```python
from build123d import *

# Parameters (mm, degrees)
F0_W     = 82.55
F0_H     = 355.6
F1_DEPTH = 4.7625
F3_D     = 9.525
F4_D     = 3
F5_D     = 6
F7_DEPTH = 4.7625


with BuildPart() as f1:
    # F0 (on Top) → F1 (new body)
    with BuildSketch(Plane.XY):
        with Locations((41.275, 0)):
            Rectangle(F0_W, F0_H)
        Polygon((82.55, 177.8), (82.55, -177.8), (139.7, -177.8), align=None)
        with Locations((-41.275, 0)):
            Rectangle(F0_W, F0_H)
        Polygon((-139.7, -177.8), (-82.55, -177.8), (-82.55, 177.8), align=None)
    extrude(amount=F1_DEPTH)

    # F3 (through all)
    with Locations(Plane.XY.offset(4.7625)):
        with Locations((-53.975, 67.945), (0, 121.92), (53.975, 67.945), (0, 13.97)):
            Hole(F3_D / 2)

    # F4 (through all)
    with Locations(Plane.XY.offset(4.7625)):
        with Locations((15.5, 83.445), (-15.5, 83.445), (-15.5, 52.445), (15.5, 52.445)):
            Hole(F4_D / 2)

    # F5 (through all)
    with Locations(Plane.XY.offset(4.7625)):
        with Locations((0, 67.945)):
            Hole(F5_D / 2)

    # F6 (on face) → F7 (join)
    with BuildSketch(Plane.XY.offset(4.7625)):
        with BuildLine():
            Line((-82.55, 177.8), (82.55, 177.8))
            ThreePointArc((82.55, 177.8), (0, 205.359059), (-82.55, 177.8))
        make_face()
    extrude(amount=-F7_DEPTH)


solid = f1.part
```
The model under review builds one solid part; all positions refer to its coordinate system, in mm. Give positions to 0.01 mm unless a question says otherwise; leave off trailing zeros. Write each loop counter-clockwise with the first axis right and the second up, starting at its lowest first coordinate (ties: lowest second). Pieces come first, ordered by that corner, then holes. Notation, with made-up numbers: M -30.75,-24 L -11.75,-24 A27 cw -11.75,-3 Z; hole C 45.5,66 d8. An arc over 180 degrees is marked long. Write item = value, one per line. Start each with the question number.
Q1. For line 1 (Y direction, x = 0, z = 1.25) (1 decimal); line 2 (Y direction, x = 15.5, z = 1.05) (3 decimals); line 3 (X direction, y = 16, z = 4.6), list the stretches that pass through material, from the lowest coordinate up.
Q2. We need section A-A (y = 13.97). State the section outline as (x, z) points.
Q3. We need section D-D (y = 121.92). State the section outline as (x, z) points.
Q4. Clearance check with a flat-ended pin moving along its axis: pin 1 (2 mm diameter, centred on y = -79.5, z = 2.5, fed in from +X). State where the tip first meets the part, or that it passes through.
Q5. We need section C-C (x = 94). State the section outline as (y, z) points, plus the area to 3 significant figures.
Q6. We need section B-B (z = 2.2). Give the number of separate pieces and of enclosed holes in the cut face, plus the area to 3 significant figures.
Q7. Mouldability with a two-part tool opening along Y and no side actions: class faces 1 (the face through (-2, -26, 0)), 2 (the face through (3.5, 17.2, 2.3)), 3 (the face through (1.24, 205.353, 2.415)) as released by +Y, released by -Y, zero draft, split by the parting line, or undercut.
Result set:
q1.line_1 = -177.8 to 9.2, 18.7 to 64.9, 70.9 to 117.2, 126.7 to 205.4
q1.line_2 = -177.8 to 50.945, 53.945 to 81.945, 84.945 to 204.482
q1.line_3 = -108.55 to -4.31, 4.31 to 108.55
q2.outline = M -108.88,0 L -4.76,0 L -4.76,4.76 L -108.88,4.76 Z; M 4.76,0 L 108.88,0 L 108.88,4.76 L 4.76,4.76 Z
q3.outline = M -91.53,0 L -4.76,0 L -4.76,4.76 L -91.53,4.76 Z; M 4.76,0 L 91.53,0 L 91.53,4.76 L 4.76,4.76 Z
q4.pin_1 = 124.06
q5.outline = M -177.8,0 L 106.56,0 L 106.56,4.76 L -177.8,4.76 Z
q5.area = 1,350 mm2
q6.separate_pieces = 1
q6.enclosed_holes = 9
q6.area = 81,800 mm2
q7.face_1 = zero draft
q7.face_2 = undercut
q7.face_3 = released by +Y
